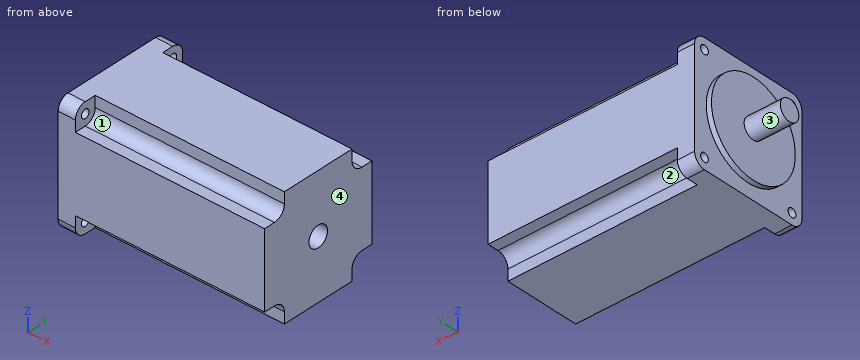
```python
from build123d import *

# Parameters (mm, degrees)
F0_R     = 9.5
F1_DEPTH = 38
F0_R_2   = 43
F2_DEPTH = 4.75
F3_DEPTH = 190
F0_R_3   = 3.96875
F4_DEPTH = 15.875


with BuildPart() as f1:
    # F0 (on Right) → F1 (new body)
    with BuildSketch(Plane.YZ):
        Circle(F0_R)
    extrude(amount=-F1_DEPTH)

    # F0 (on Right) → F2 (join)
    with BuildSketch(Plane.YZ):
        Circle(F0_R_2)
        Circle(F0_R, mode=Mode.SUBTRACT)
    extrude(amount=-F2_DEPTH)

    # F0 (on Right) → F3 (join)
    with BuildSketch(Plane.YZ):
        with BuildLine():
            Line((-34.68, -55), (34.68, -55))
            Line((34.68, -55), (34.68, -44.84))
            ThreePointArc((34.68, -44.84), (37.6557951031, -37.6557951031), (44.84, -34.68))
            Line((44.84, -34.68), (55, -34.68))
            Line((55, -34.68), (55, 34.68))
            Line((55, 34.68), (44.84, 34.68))
            ThreePointArc((44.84, 34.68), (37.6557951031, 37.6557951031), (34.68, 44.84))
            Line((34.68, 44.84), (34.68, 55))
            Line((34.68, 55), (-34.68, 55))
            Line((-34.68, 55), (-34.68, 44.84))
            ThreePointArc((-34.68, 44.84), (-37.6557951031, 37.6557951031), (-44.84, 34.68))
            Line((-44.84, 34.68), (-55, 34.68))
            Line((-55, 34.68), (-55, -34.68))
            Line((-55, -34.68), (-44.84, -34.68))
            ThreePointArc((-44.84, -34.68), (-37.6557951031, -37.6557951031), (-34.68, -44.84))
            Line((-34.68, -44.84), (-34.68, -55))
        make_face()
        Circle(F0_R_2, mode=Mode.SUBTRACT)
        Circle(F0_R_2)
        Circle(F0_R, mode=Mode.SUBTRACT)
    extrude(amount=F3_DEPTH)

    # F0 (on Right) → F4 (join)
    with BuildSketch(Plane.YZ):
        with BuildLine():
            Line((-55, 44.84), (-55, 34.68))
            Line((-55, 34.68), (-44.84, 34.68))
            ThreePointArc((-44.84, 34.68), (-37.6557951031, 37.6557951031), (-34.68, 44.84))
            Line((-34.68, 44.84), (-34.68, 55))
            Line((-34.68, 55), (-44.84, 55))
            ThreePointArc((-44.84, 55), (-52.0242048969, 52.0242048969), (-55, 44.84))
        make_face()
        with Locations((-44.84, 44.84)):
            Circle(F0_R_3, mode=Mode.SUBTRACT)
        with BuildLine():
            Line((44.84, 34.68), (55, 34.68))
            Line((55, 34.68), (55, 44.84))
            ThreePointArc((55, 44.84), (52.0242048969, 52.0242048969), (44.84, 55))
            Line((44.84, 55), (34.68, 55))
            Line((34.68, 55), (34.68, 44.84))
            ThreePointArc((34.68, 44.84), (37.6557951031, 37.6557951031), (44.84, 34.68))
        make_face()
        with Locations((44.84, 44.84)):
            Circle(F0_R_3, mode=Mode.SUBTRACT)
        with BuildLine():
            Line((34.68, -55), (44.84, -55))
            ThreePointArc((44.84, -55), (52.0242048969, -52.0242048969), (55, -44.84))
            Line((55, -44.84), (55, -34.68))
            Line((55, -34.68), (44.84, -34.68))
            ThreePointArc((44.84, -34.68), (37.6557951031, -37.6557951031), (34.68, -44.84))
            Line((34.68, -44.84), (34.68, -55))
        make_face()
        with Locations((44.84, -44.84)):
            Circle(F0_R_3, mode=Mode.SUBTRACT)
        with BuildLine():
            Line((-44.84, -55), (-34.68, -55))
            Line((-34.68, -55), (-34.68, -44.84))
            ThreePointArc((-34.68, -44.84), (-37.6557951031, -37.6557951031), (-44.84, -34.68))
            Line((-44.84, -34.68), (-55, -34.68))
            Line((-55, -34.68), (-55, -44.84))
            ThreePointArc((-55, -44.84), (-52.0242048969, -52.0242048969), (-44.84, -55))
        make_face()
        with Locations((-44.84, -44.84)):
            Circle(F0_R_3, mode=Mode.SUBTRACT)
    extrude(amount=F4_DEPTH)


solid = f1.part
```
Could you check a few things on this model? Use its own coordinates, in mm. Face numbers are marked on the shaded views. A direction names the side the tool comes from. Coordinates: 2 decimals unless noted, no trailing zeros. Write each loop counter-clockwise with the first axis right and the second up, starting at its lowest first coordinate (ties: lowest second). Pieces come first, ordered by that corner, then holes. Notation, with made-up numbers: (33, 10) -> (40, 10) arc R26 ccw to (40, 37) -> close; hole circle Ø9 at (28.5, -1.5). An arc over 180 degrees is marked (long way). One line per question, with ' | ' between items. Start each with the question number.
1. If we section it at B-B (z = 0): Please give me the cut outline in (x, y), and give its area (3 significant figures).
2. If we section it at C-C (x = 8.5): Please give me the cut outline in (y, z), and give its area (3 significant figures).
3. If we section it at A-A (x = 116.5): Please give me the cut outline in (y, z), and give its area (3 significant figures).
4. Will these pins go through, and if not, where does the flat tip stop? P1, Ø3, axis at x = 60.5, z = 49.5, coming from the -Y side; P2, Ø6, axis at y = 42.5, z = -43, coming from the +X side (3 decimals); P3, Ø9, axis at y = 44.84, z = 44.84, coming from the -X side; P4, Ø5, axis at y = -44.84, z = 44.84, coming from the -X side.
5. For the marked faces 1, 2, 3 and 4, which set-ups out of +Z, -Z, +X, -X, +Y, -Y let a thin tool reach every point of the face, with its end or its side?
6. Please list where these lines run through material, in increasing order: line 1 along Z through (x, y) = (8, -44); line 2 along Z through (x, y) = (133, 0); line 3 along X through (y, z) = (38, 31).
Return value:
1) outline: (-38, -9.5) -> (-4.75, -9.5) -> (-4.75, -43) -> (0, -43) -> (0, -55) -> (190, -55) -> (190, -9.5) -> (0, -9.5) -> (0, 9.5) -> (190, 9.5) -> (190, 55) -> (0, 55) -> (0, 43) -> (-4.75, 43) -> (-4.75, 9.5) -> (-38, 9.5) -> close | area: 18,300 mm²
2) outline: (-55, -44.84) arc R10.16 ccw to (-44.84, -55) -> (44.84, -55) arc R10.16 ccw to (55, -44.84) -> (55, 44.84) arc R10.16 ccw to (44.84, 55) -> (-44.84, 55) arc R10.16 ccw to (-55, 44.84) -> close; hole circle Ø7.94 at (-44.84, -44.84); hole circle Ø7.94 at (-44.84, 44.84); hole circle Ø19 at (0, 0); hole circle Ø7.94 at (44.84, -44.84); hole circle Ø7.94 at (44.84, 44.84) | area: 11,500 mm²
3) outline: (-55, -34.68) -> (-44.84, -34.68) arc R10.16 cw to (-34.68, -44.84) -> (-34.68, -55) -> (34.68, -55) -> (34.68, -44.84) arc R10.16 cw to (44.84, -34.68) -> (55, -34.68) -> (55, 34.68) -> (44.84, 34.68) arc R10.16 cw to (34.68, 44.84) -> (34.68, 55) -> (-34.68, 55) -> (-34.68, 44.84) arc R10.16 cw to (-44.84, 34.68) -> (-55, 34.68) -> close; hole circle Ø19 at (0, 0) | area: 10,300 mm²
4) P1: stops at y = -34.68 | P2: stops at x = 15.875 | P3: stops at x = 0 | P4: passes through
5) face 1: +Z, +X, -Y | face 2: -Z, +X, +Y | face 3: -X | face 4: +Z, -Z, +X, +Y, -Y
6) line 1: z = -55 to -48.72, -40.96 to 40.96, 48.72 to 55 | line 2: z = -55 to -9.5, 9.5 to 55 | line 3: x = 0 to 190
